CAD build for the part. Positions are in the model's coordinates, mm. A direction names the side the tool comes from. Round coordinates to 2 decimals unless told otherwise and drop trailing zeros. Order: outer loops, then holes, each group sorted by start corner. A loop starts at its lowest first (then second) coordinate and runs counter-clockwise, first axis right, second up.
Autodesk Inventor part; units mm, degrees
ref_plane "YZ Plane" through (0, 0, 0) normal (1, 0, 0) x (0, 1, 0)
ref_plane "XZ Plane" through (0, 0, 0) normal (0, 1, 0) x (-1, 0, 0)
ref_plane "XY Plane" through (0, 0, 0) normal (0, 0, 1) x (1, 0, 0)
sketch "Sketch1" plane through (0, 0, 0) normal (0, 1, 0) x (-1, 0, 0)
  line L0 (-15, -15) -> (15, -15)
  line L1 (15, -15) -> (15, 15)
  line L2 (15, 15) -> (-15, 15)
  line L3 (-15, 15) -> (-15, -15)
  line L4 (-15, -15) -> (15, 15) construction
  line L5 (15, -15) -> (-15, 15) construction
  line L6 (-2.45, -12.65) -> (2.45, -12.65) construction
  line L7 (2.45, -12.65) -> (2.45, 12.65) construction
  line L8 (2.45, 12.65) -> (-2.45, 12.65) construction
  line L9 (-2.45, 12.65) -> (-2.45, -12.65) construction
  line L10 (-2.45, -12.65) -> (2.45, 12.65) construction
  line L11 (2.45, -12.65) -> (-2.45, 12.65) construction
  line L12 (-12.65, -2.45) -> (12.65, -2.45) construction
  line L13 (12.65, -2.45) -> (12.65, 2.45) construction
  line L14 (12.65, 2.45) -> (-12.65, 2.45) construction
  line L15 (-12.65, 2.45) -> (-12.65, -2.45) construction
  line L16 (-12.65, -2.45) -> (12.65, 2.45) construction
  line L17 (12.65, -2.45) -> (-12.65, 2.45) construction
  line L18 (-12.85, -2.65) -> (12.85, -2.65)
  line L19 (12.85, -2.65) -> (12.85, 2.65)
  line L20 (12.85, 2.65) -> (-12.85, 2.65)
  line L21 (-12.85, 2.65) -> (-12.85, -2.65)
  line L22 (-12.85, -2.65) -> (12.85, 2.65) construction
  line L23 (12.85, -2.65) -> (-12.85, 2.65) construction
  line L24 (-2.65, -12.85) -> (2.65, -12.85)
  line L25 (2.65, -12.85) -> (2.65, 12.85)
  line L26 (2.65, 12.85) -> (-2.65, 12.85)
  line L27 (-2.65, 12.85) -> (-2.65, -12.85)
  line L28 (-2.65, -12.85) -> (2.65, 12.85) construction
  line L29 (2.65, -12.85) -> (-2.65, 12.85) construction
  point P0 (0, 0)
  point P1 (0, 0)
  dimension "d0" = 30
  dimension "d1" = 4.9
  dimension "d2" = 10.2
  dimension "d3" = 0.2
  dimension "d4" = 0.2
extrude "Extrusion1" add sketch "Sketch1" along normal blind 1.9
sketch "Sketch2" plane through (0, 1.9, 0) normal (0, 1, 0) x (1, 0, 0)
  line L0 (15, 15) -> (-15, 15)
  line L1 (-15, 15) -> (-15, -15)
  line L2 (-15, -15) -> (15, -15)
  line L3 (15, -15) -> (15, 15)
  circle A0 centre (0, 0) radius 1.5
  dimension "d7" = 3
extrude "Extrusion2" add sketch "Sketch2" along normal blind 2
sketch "Sketch3" plane through (0, 3.9, 0) normal (0, 1, 0) x (1, 0, 0)
  circle A0 centre (0, 0) radius 1.5
  line L0 (15, 15) -> (-15, 15)
  line L1 (-15, 15) -> (-15, -15)
  line L2 (-15, -15) -> (15, -15)
  line L3 (15, -15) -> (15, 15)
  circle A1 centre (0, 0) radius 2.75
  dimension "d10" = 5.5
extrude "Extrusion3" add sketch "Sketch3" along normal blind 0.5 contours L3 L2 L1 L0
chamfer "Chamfer1" distance 2 angle 45 1 edges at (-2.65, 0.95, -2.65)
fillet "Fillet1" radius 2.45 1 edges at (-12.85, 0.95, -2.65)
fillet "Fillet2" radius 2.45 1 edges at (-2.65, 0.95, -12.85)
chamfer "Chamfer2" distance 2 angle 45 1 edges at (2.65, 0.95, -2.65)
chamfer "Chamfer3" distance 2 angle 45 1 edges at (2.65, 0.95, 2.65)
fillet "Fillet3" radius 2.45 1 edges at (12.85, 0.95, -2.65)
fillet "Fillet4" radius 2.45 1 edges at (2.65, 0.95, -12.85)
fillet "Fillet5" radius 2.45 1 edges at (12.85, 0.95, 2.65)
fillet "Fillet6" radius 2.45 1 edges at (2.65, 0.95, 12.85)
chamfer "Chamfer4" distance 2 angle 45 1 edges at (-2.65, 0.95, 2.65)
fillet "Fillet7" radius 2.45 2 edges at (-2.65, 0.95, 12.85) (-12.85, 0.95, 2.65)
sketch "Sketch4" plane through (0, 0, 0) normal (0, -1, 0) x (1, 0, 0)
  line L0 (15, -15) -> (-15, -15)
  line L1 (-10.4, 2.65) -> (-4.65, 2.65)
  line L2 (0, 0) -> (0, -74.1645) construction
  line L3 (-15, -15) -> (-10, -70)
  line L4 (15, -15) -> (10, -70)
  line L5 (-10, -70) -> (10, -70)
  arc A0 (-10, -70) -> (10, -70) centre (0, -70) ccw
  dimension "d32" = 70
  dimension "d33" = 20
extrude "Extrusion4" add sketch "Sketch4" against normal up to surface (4.4 mm away)
equation "\"d0\" = BackLowerLegKneeWidth"
equation "\"d1\" = ServoArmWidth"
equation "\"d2\" = ServoArmLength"
equation "\"d3\" = ServoArmSpacing"
equation "\"d4\" = ServoArmSpacing"
equation "\"d5\" = ServoArmThickness"
equation "\"d7\" = ServoArmHoleRequired"
equation "\"d8\" = MinimalThickness"
equation "\"d10\" = ServoArmHeadScrewTrace"
equation "\"d11\" = ServoArmHeadScrewThickness"
equation "\"d13\" = ServoArmInternFillet"
equation "\"d16\" = ServoArmExternFillet"
equation "\"d17\" = ServoArmExternFillet"
equation "\"d18\" = ServoArmInternFillet"
equation "\"d21\" = ServoArmInternFillet"
equation "\"d24\" = ServoArmExternFillet"
equation "\"d25\" = ServoArmExternFillet"
equation "\"d26\" = ServoArmExternFillet"
equation "\"d27\" = ServoArmExternFillet"
equation "\"d28\" = ServoArmInternFillet"
equation "\"d31\" = ServoArmExternFillet"
equation "\"d32\" = BackLowerLegLength"
equation "\"d33\" = BackLowerLegFootWidth"
equation "\"d34\" = ServoArmHoleRequired"
equation "\"BackLowerLegLength\" = 70"
equation "\"BackLowerLegFootWidth\" = 20"
equation "\"BackLowerLegKneeWidth\" = 30"
properties part number "BackLowerLeg" material "PC/ABS Plastic"
1. Mould opens along Z. For faces 1 (the face through (1.913, 0.963, 12.151)), 2 (the face through (0, 2, 15)), 3 (the face through (0, 0, -32)), 4 (the face through (-12.535, 2.169, -42.115)) say: released by +Z, released by -Z, zero draft, split by the parting line, or undercut.
2. Pin check, flat tips, straight feed: P1, Ø1, axis at x = 5.5, y = 1, coming from the -Z side; P2, Ø2, axis at y = 1.5, z = -33.5, coming from the -X side; P3, Ø1, axis at y = 4, z = -36, coming from the +X side. Stop position of each tip, or through.
3. Cut at B-B, the plane z = -38. Write the cut outline in (x, y).
4. Tool access for faces 5 (the face through (2.65, 1, 8)), 6 (the face through (0, 2, -80)), 7 (the face through (-0.596, 4.147, -2.685)): list every direction of +Z, -Z, +X, -X, +Y, -Y with a clear straight run to the whole face (end or side of a thin tool).
5. Cut at A-A, the plane y = 2.65. Write the cut outline in (x, z).
6. Cut at C-C, the plane z = -24. Write the cut outline in (x, y).
7. Drill centre lines: line 1 (X direction, y = 4.15, z = 0); line 2 (Z direction, x = 0, y = 4.25); line 3 (Z direction, x = 0, y = 2.5). Where is each one in solid material? Low to high.
Outcome:
1. face 1: undercut
1. face 2: released by +Z
1. face 3: zero draft
1. face 4: released by -Z
2. P1: stops at z = -78.66
2. P2: stops at x = -13.41
2. P3: stops at x = 13.14
3. outline: (-12.91, 0) - (12.91, 0) - (12.91, 4.4) - (-12.91, 4.4) - close
4. face 5: -Y
4. face 6: -Z, +Y, -Y
4. face 7: +Y
5. outline: (-15, -15) - (-10, -70) arc R10 ccw to (10, -70) - (15, -15) - (15, 15) - (-15, 15) - close; hole circle Ø3 at (0, 0)
6. outline: (-14.18, 0) - (14.18, 0) - (14.18, 4.4) - (-14.18, 4.4) - close
7. line 1: x = -15 to -2.75, 2.75 to 15
7. line 2: z = -80 to -2.75, 2.75 to 15
7. line 3: z = -80 to -1.5, 1.5 to 15
